from build123d import *

# Parameters (mm, degrees)
BOSS_EXTRUDE1_DEPTH = 25.4
CUT_EXTRUDE1_REACH  = 52.064
SKETCH2_R           = 3.175
FILLET1_R           = 2.54
CUT_EXTRUDE2_REACH  = 47.354
SKETCH3_R           = 2.921
CUT_EXTRUDE3_REACH  = 49.286
SKETCH4_R           = 2.921


with BuildPart() as part:
    # Sketch1 → Boss-Extrude1 (new body)
    with BuildSketch(Plane(origin=(0, 0, 0), x_dir=(1, 0, 0), z_dir=(0, 1, 0))):
        with BuildLine():
            Line((0, 0), (0, 31.75))
            Line((0, 31.75), (3.81, 31.75))
            Line((3.81, 31.75), (3.81, 13.44041666))
            ThreePointArc((3.81, 13.44041666), (12.879954362, 16.776213121), (20.638087116, 11.014009869))
            Line((20.638087116, 11.014009869), (28.987665935, 11.744503361))
            Line((28.987665935, 11.744503361), (29.209041521, 9.214168828))
            Line((29.209041521, 9.214168828), (19.087703389, 8.328666482))
            Line((19.087703389, 8.328666482), (18.336065337, 9.940559485))
            ThreePointArc((18.336065337, 9.940559485), (9.780730142, 14.159583904), (3.81, 6.72020833))
            ThreePointArc((3.81, 6.72020833), (9.780730142, -0.719167244), (18.336065337, 3.499857176))
            Line((18.336065337, 3.499857176), (19.087703389, 5.111750178))
            Line((19.087703389, 5.111750178), (29.209041521, 4.226247832))
            Line((29.209041521, 4.226247832), (28.987665935, 1.695913299))
            Line((28.987665935, 1.695913299), (20.638087116, 2.426406791))
            ThreePointArc((20.638087116, 2.426406791), (12.879954362, -3.335796461), (3.81, 0))
            Line((3.81, 0), (0, 0))
        make_face()
    extrude(amount=BOSS_EXTRUDE1_DEPTH)

    # Sketch2 → Cut-Extrude1 (cut, up to next)
    with BuildSketch(Plane.ZY, mode=Mode.PRIVATE) as cut_extrude1_sk1:
        with Locations((-21.59, 12.7)):
            Circle(SKETCH2_R)
    cut_extrude1_tool1 = extrude(cut_extrude1_sk1.sketch, amount=-CUT_EXTRUDE1_REACH, mode=Mode.PRIVATE) & part.part
    add(cut_extrude1_tool1.solids().sort_by_distance((0, 12.7, -21.59))[0], mode=Mode.SUBTRACT)

    # Fillet1
    fillet1_edges = [part.edges().sort_by_distance(p)[0] for p in [
        (1.905, 0, -31.75),
        (1.905, 0, 0),
        (1.905, 25.4, 0),
        (1.905, 25.4, -31.75),
    ]]
    fillet(fillet1_edges, radius=FILLET1_R)

    # Sketch3 → Cut-Extrude2 (cut, up to next)
    with BuildSketch(Plane(origin=(-0.799511913, 0, -9.138462981), x_dir=(-0.996194698091745, 0, 0.08715574274766381), z_dir=(-0.08715574274766381, 0, -0.9961946980917451)), mode=Mode.PRIVATE) as cut_extrude2_sk1:
        with Locations((-25.710223601, 19.05)):
            Circle(SKETCH3_R)
    cut_extrude2_tool1 = extrude(cut_extrude2_sk1.sketch, amount=-CUT_EXTRUDE2_REACH, mode=Mode.PRIVATE) & part.part
    # Sketch3 → Cut-Extrude2 (cut, up to next)
    with BuildSketch(Plane(origin=(-0.799511913, 0, -9.138462981), x_dir=(-0.996194698091745, 0, 0.08715574274766381), z_dir=(-0.08715574274766381, 0, -0.9961946980917451)), mode=Mode.PRIVATE) as cut_extrude2_sk2:
        with Locations((-25.710223601, 6.35)):
            Circle(SKETCH3_R)
    cut_extrude2_tool2 = extrude(cut_extrude2_sk2.sketch, amount=-CUT_EXTRUDE2_REACH, mode=Mode.PRIVATE) & part.part
    add(cut_extrude2_tool1.solids().sort_by_distance((24.812877, 19.05, -11.379257))[0], mode=Mode.SUBTRACT)
    add(cut_extrude2_tool2.solids().sort_by_distance((24.812877, 6.35, -11.379257))[0], mode=Mode.SUBTRACT)

    # Sketch4 → Cut-Extrude3 (cut, up to next)
    with BuildSketch(Plane(origin=(0.367440017, 0, -4.199858614), x_dir=(0.9961946980917455, 0, 0.0871557427476594), z_dir=(-0.0871557427476594, 0, 0.9961946980917455)), mode=Mode.PRIVATE) as cut_extrude3_sk1:
        with Locations((24.538814104, 19.05)):
            Circle(SKETCH4_R)
    cut_extrude3_tool1 = extrude(cut_extrude3_sk1.sketch, amount=-CUT_EXTRUDE3_REACH, mode=Mode.PRIVATE) & part.part
    # Sketch4 → Cut-Extrude3 (cut, up to next)
    with BuildSketch(Plane(origin=(0.367440017, 0, -4.199858614), x_dir=(0.9961946980917455, 0, 0.0871557427476594), z_dir=(-0.0871557427476594, 0, 0.9961946980917455)), mode=Mode.PRIVATE) as cut_extrude3_sk2:
        with Locations((24.538814104, 6.35)):
            Circle(SKETCH4_R)
    cut_extrude3_tool2 = extrude(cut_extrude3_sk2.sketch, amount=-CUT_EXTRUDE3_REACH, mode=Mode.PRIVATE) & part.part
    add(cut_extrude3_tool1.solids().sort_by_distance((24.812877, 19.05, -2.06116))[0], mode=Mode.SUBTRACT)
    add(cut_extrude3_tool2.solids().sort_by_distance((24.812877, 6.35, -2.06116))[0], mode=Mode.SUBTRACT)


solid = part.part
Here's how the part is built. I have some questions about the finished solid (model axes, mm). A direction names the side the tool comes from. Coordinates: 2 decimals unless noted, no trailing zeros. Write each loop counter-clockwise with the first axis right and the second up, starting at its lowest first coordinate (ties: lowest second). Pieces come first, ordered by that corner, then holes.
Item 1: If I drill on line 1 (Y direction, x = 2.3, z = -21.59) (3 decimals); line 2 (Z direction, x = 11.75, y = 10.25); line 3 (X direction, y = 8.75, z = -2), over which ranges is the centre line in solid material (lowest first)?
Item 2: Will these pins go through, and if not, where does the flat tip stop? pin 1 (8 mm diameter, centred on x = 25.5, y = 10.5, fed in from -Z); pin 2 (12 mm diameter, centred on x = 25.5, z = -20, fed in from +Y); pin 3 (1 mm diameter, centred on y = 18.5, z = -21, fed in from +X); pin 4 (1.9 mm diameter, centred on x = 1, y = 11, fed in from +Z).
Item 3: I want a section at D-D on x = 10.5. Write out the boundary of the cut face in (y, z), and give its area (3 significant figures).
Item 4: I want a section at C-C on y = 7. Write out the boundary of the cut face in (x, z), and give its area (3 significant figures).
Item 5: If we mould it in two halves opening along Y, with no side actions, what happens to faces 1 (the cylindrical face through (27.07, 8.32, -10.32)), 2 (the flat face through (24.754, 12.522, -11.374)), 3 (the flat face through (6, 25.4, -13))? For each: +Y half, -Y half, draft (parallel to the pull), parting line (faces both ways), or undercut.
Item 6: I want a section at A-A on z = -21.59. Write out the boundary of the cut face in (x, y) (3 decimals).
Item 7: On a 3-axis mill with a long thin cutter (end or side, diameter ignored), from which of +Z, -Z, +X, -X, +Y, -Y can I reach the whole of each face in a straight line? I mean faces 4 (the cylindrical face through (1.455, 0.764, -0.724)), 5 (the flat face through (24.078, 12.522, -4.675)), 6 (the flat face through (18.707, 12.522, -4.295)), 7 (the flat face through (24.871, 12.522, -2.056)). Say none if no direction works.
Findings below:
1. line 1: y = 0 to 9.525, 15.875 to 25.4
1. line 2: z = -16.88 to -14.33, 0.89 to 3.43
1. line 3: x = 0 to 5.45, 17.41 to 20.43, 26.48 to 29.01
2. pin 1: stops at z = -11.74
2. pin 2: passes through
2. pin 3: stops at x = 3.81
2. pin 4: stops at z = 0
3. outline: (0, -16.84) - (25.4, -16.84) - (25.4, -14.28) - (0, -14.28) - close; (0, 0.84) - (25.4, 0.84) - (25.4, 3.4) - (0, 3.4) - close
3. area: 130 mm2
4. outline: (0, -31.75) - (3.81, -31.75) - (3.81, -13.44) arc R10.16 ccw to (20.64, -11.01) - (21.98, -11.13) - (22.2, -8.6) - (19.09, -8.33) - (18.34, -9.94) arc R7.62 cw (long way) to (18.34, -3.5) - (19.09, -5.11) - (22.2, -4.84) - (21.98, -2.31) - (20.64, -2.43) arc R10.16 ccw to (3.81, 0) - (0, 0) - close; (27.65, -11.63) - (28.99, -11.74) - (29.21, -9.21) - (27.87, -9.1) - close; (27.65, -1.81) - (27.87, -4.34) - (29.21, -4.23) - (28.99, -1.7) - close
4. area: 242 mm2
5. face 1: undercut
5. face 2: draft
5. face 3: +Y half
6. outline: (0, 0) - (3.81, 0) - (3.81, 9.525) - (0, 9.525) - close; (0, 15.875) - (3.81, 15.875) - (3.81, 25.4) - (0, 25.4) - close
7. face 4: +Z, -X, -Y
7. face 5: +X, +Y, -Y
7. face 6: +Y, -Y
7. face 7: +Z, +Y, -Y
